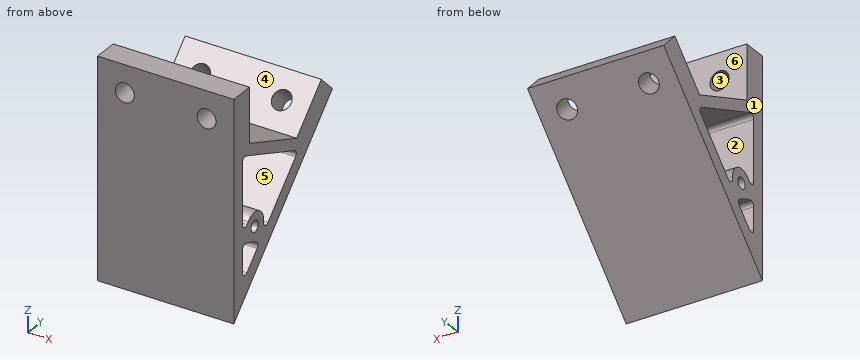
```python
from build123d import *

# Parameters (mm, degrees)
BOSS_EXTRUDE1_DEPTH      = 25
BOSS_EXTRUDE1_DEPTH_BACK = 25
SKETCH1_R                = 2.1
SKETCH2_R                = 3.5
CUT_EXTRUDE1_DEPTH       = 9
SKETCH3_R                = 3.5
CUT_EXTRUDE2_DEPTH       = 9
SKETCH4_R                = 3.5
CUT_EXTRUDE3_DEPTH       = 9
SKETCH5_R                = 3.5
CUT_EXTRUDE4_DEPTH       = 9


with BuildPart() as part:
    # Sketch1 → Boss-Extrude1 (new, two sides: drawn at the far end of the back side and taken through both)
    with BuildSketch(Plane(origin=(0, 0, 0), x_dir=(0, 0, -1), z_dir=(1, 0, 0)).offset(-BOSS_EXTRUDE1_DEPTH_BACK)):
        Polygon((-80, 0), (0, 0), (-56.568542495, 56.568542495), (-62.932503526, 50.204581464), (-48.790367902, 36.062445841), (-60, 9), (-80, 9), align=None)
        with Locations((-28.970562748, 12)):
            Circle(SKETCH1_R, mode=Mode.SUBTRACT)
        with BuildLine():
            Line((-23.933031567, 5), (-15.692388155, 5))
            ThreePointArc((-15.692388155, 5), (-14.306568857, 5.925974851), (-14.631727984, 7.560660172))
            Line((-14.631727984, 7.560660172), (-20.458742822, 13.38767501))
            ThreePointArc((-20.458742822, 13.38767501), (-21.717716442, 13.813847638), (-22.820979835, 13.072600329))
            ThreePointArc((-22.820979835, 13.072600329), (-24.298031724, 10.064574227), (-25.38059396, 6.893145161))
            ThreePointArc((-25.38059396, 6.893145161), (-25.124609878, 5.588879191), (-23.933031567, 5))
        make_face(mode=Mode.SUBTRACT)
        with BuildLine():
            Line((-55.082376804, 5), (-32.755922357, 5))
            ThreePointArc((-32.755922357, 5), (-31.361417837, 5.947408702), (-31.728467606, 7.592857143))
            Line((-31.728467606, 7.592857143), (-32.463908902, 8.284285714))
            ThreePointArc((-32.463908902, 8.284285714), (-33.682348364, 13.951685505), (-28.813324734, 17.097575522))
            Line((-28.813324734, 17.097575522), (-27.804375375, 17.066453827))
            ThreePointArc((-27.804375375, 17.066453827), (-26.381324244, 17.970418197), (-26.697468729, 19.626400917))
            Line((-26.697468729, 19.626400917), (-42.484656068, 35.413588256))
            ThreePointArc((-42.484656068, 35.413588256), (-43.837951723, 35.824106005), (-44.931135539, 34.926953233))
            Line((-44.931135539, 34.926953233), (-56.468196103, 7.074025149))
            ThreePointArc((-56.468196103, 7.074025149), (-56.329581223, 5.66664465), (-55.082376804, 5))
        make_face(mode=Mode.SUBTRACT)
    extrude(amount=BOSS_EXTRUDE1_DEPTH + BOSS_EXTRUDE1_DEPTH_BACK)

    # Sketch2 → Cut-Extrude1 (cut)
    with BuildSketch(Plane(origin=(0, -6.363961031, 6.363961031), x_dir=(1, 0, 0), z_dir=(0, -0.7071067811865467, 0.7071067811865485))):
        with Locations(Location((-15, 70, 0), (0, 0, 270))):
            Circle(SKETCH2_R)
    extrude(amount=-CUT_EXTRUDE1_DEPTH, mode=Mode.SUBTRACT)

    # Sketch3 → Cut-Extrude2 (cut)
    with BuildSketch(Plane(origin=(0, -6.363961031, 6.363961031), x_dir=(1, 0, 0), z_dir=(0, -0.7071067811865467, 0.7071067811865485))):
        with Locations(Location((15, 70, 0), (0, 0, 270))):
            Circle(SKETCH3_R)
    extrude(amount=-CUT_EXTRUDE2_DEPTH, mode=Mode.SUBTRACT)

    # Sketch4 → Cut-Extrude3 (cut)
    with BuildSketch(Plane(origin=(0, 0, 0), x_dir=(1, 0, 0), z_dir=(0, 1, 0))):
        with Locations(Location((-15, -70, 0), (0, 0, 270))):
            Circle(SKETCH4_R)
    extrude(amount=CUT_EXTRUDE3_DEPTH, mode=Mode.SUBTRACT)

    # Sketch5 → Cut-Extrude4 (cut)
    with BuildSketch(Plane(origin=(0, 0, 0), x_dir=(1, 0, 0), z_dir=(0, 1, 0))):
        with Locations(Location((15, -70, 0), (0, 0, 270))):
            Circle(SKETCH5_R)
    extrude(amount=CUT_EXTRUDE4_DEPTH, mode=Mode.SUBTRACT)


solid = part.part
```
Build history of the part. All positions in model axes, mm. Face numbers are marked on the shaded views. A direction names the side the tool comes from. Coordinates: 2 decimals unless noted, no trailing zeros. Write each loop counter-clockwise with the first axis right and the second up, starting at its lowest first coordinate (ties: lowest second). Pieces come first, ordered by that corner, then holes.
1. Band-saw the part on D-D, the plane x = -15. Give the number of separate pieces and of enclosed holes in the cut face, and give its area (3 significant figures).
Answer block:
separate pieces: 3
enclosed holes: 3
area: 1,010 mm2
2. Band-saw the part on B-B, the plane x = -20. Give the cut face in (y, z).
Answer block:
outline: (0, 0) - (56.57, 56.57) - (50.2, 62.93) - (36.06, 48.79) - (9, 60) - (9, 80) - (0, 80) - close; hole (5, 15.69) arc R1.5 ccw to (7.56, 14.63) - (13.39, 20.46) arc R1.5 ccw to (13.07, 22.82) arc R26.3 ccw to (6.89, 25.38) arc R1.5 ccw to (5, 23.93) - close; hole (5, 32.76) arc R1.5 ccw to (7.59, 31.73) - (8.28, 32.46) arc R5.1 cw to (17.1, 28.81) - (17.07, 27.8) arc R1.5 ccw to (19.63, 26.7) - (35.41, 42.48) arc R1.5 ccw to (34.93, 44.93) - (7.07, 56.47) arc R1.5 ccw to (5, 55.08) - close; hole circle Ø4.2 at (12, 28.97)
3. 3-axis set-ups, long thin cutter, end or side, ignore diameter. For the marked faces 1 and 2: which of +Z, -Z, +X, -X, +Y, -Y reach the whole face in a straight line?
Answer block:
face 1: +Z, -Z, -X, +Y, -Y
face 2: +X, -X
4. Pull direction Z, two halves, no side cores. Call the marked faces 3, 4, 5 and 6: released by +Z, released by -Z, zero draft, split by the parting line, or undercut.
Answer block:
face 3: undercut
face 4: released by +Z
face 5: undercut
face 6: zero draft
5. Band-saw the part on A-A, the plane z = 70. Give the cut face in (x, y), and give its area (3 significant figures).
Answer block:
outline: (-25, 0) - (-18.5, 0) - (-18.5, 9) - (-25, 9) - close; (-11.5, 0) - (11.5, 0) - (11.5, 9) - (-11.5, 9) - close; (18.5, 0) - (25, 0) - (25, 9) - (18.5, 9) - close
area: 324 mm2
6. Drop flat-ended pins along their axis: pin 1 (18 mm diameter, centred on x = -2, z = 46, fed in from +Y); pin 2 (6 mm diameter, centred on x = -3.5, y = 29, fed in from +Z); pin 3 (3.5 mm diameter, centred on y = 12, z = 28.97, fed in from -X); pin 4 (6 mm diameter, centred on x = -14, y = 30, fed in from +Z). Give the stop position or say it passes through.
Answer block:
pin 1: stops at y = 55
pin 2: stops at z = 52.96
pin 3: passes through
pin 4: stops at z = 52.54
7. Drill centre lines: probe 1 along X at (y, z) = (3, 70); probe 2 along Y at (x, z) = (7, 70.5); probe 3 along Z at (x, y) = (18, 19). Where is each one in solid material? Low to high.
Answer block:
probe 1: x = -25 to -18.5, -11.5 to 11.5, 18.5 to 25
probe 2: y = 0 to 9
probe 3: z = 19 to 26.32, 51.53 to 55.86
8. Band-saw the part on C-C, the plane y = 4. Give the cut face in (x, z).
Answer block:
outline: (-25, 4) - (25, 4) - (25, 80) - (-25, 80) - close; hole circle Ø7 at (-15, 70); hole circle Ø7 at (15, 70)
